Source: CAD feature listing. Evaluate the final solid. Frame: model axes, mm. A direction names the side the tool comes from. Coordinates: 2 decimals unless noted, no trailing zeros.
Item 1: Section query B-B, the plane z = 0. State how many separate pieces and enclosed holes the cut face has, then the cut area to 3 significant figures.
Item 2: Pull-direction query (Z, two-part tool) for faces 3 (the flat face through (44, 4, 26)), 4 (the flat face through (44, 4, -26)), 5 (the cylindrical face through (-36.926, 1.186, 22.404)); classes: +Z half, -Z half, draft (parallel to the pull), parting line (faces both ways), or undercut.
Item 3: Reachability of faces 1 (the cylindrical face through (-37.136, 1.214, -20.813)), 2 (the flat face through (38, 3.4, 24)) from +Z, -Z, +X, -X, +Y, -Y: full face, straight path, thin tool, end or side. Return the list, or none.
Item 4: Pin query (flat end, axial travel): pin 1 Ø15.5 at (x, z) = (-24, 1) entering from -Y; pin 2 Ø5 at (x, z) = (-40, 22) entering from +Y; pin 3 Ø9.5 at (x, z) = (-21, 0) entering from -Y; pin 4 Ø12 at (x, z) = (-23, 1) entering from -Y. Return the tip coordinate at first contact, or that it passes through.
Item 5: Line query: probe 1 along Z at (x, y) = (40, 2.75); probe 2 along Z at (x, y) = (40, 0.7); probe 3 along X at (y, z) = (3.45, 0). Output: solid intervals per line, ascending.
```python
from build123d import *

# Parameters (mm, degrees)
SKETCH1_W           = 96
SKETCH1_H           = 60
BOSS_EXTRUDE1_DEPTH = 8
CHAMFER1_SIZE       = 8
HOLE4_D             = 24.1
HOLE4_DEPTH         = 5.2
SKETCH10_R          = 10
CUT_EXTRUDE1_DEPTH  = 0.2
CHAMFER2_SIZE       = 0.2
SKETCH11_R          = 3.1
CUT_EXTRUDE2_DEPTH  = 2.2
CHAMFER3_SIZE       = 0.2
SKETCH15_R          = 8
CUT_EXTRUDE3_DEPTH  = 57.860882863
CHAMFER4_SIZE       = 0.4


# Read off the part's stored shape, not the designer's step: CBORE for M4 SHCS1, Sketch-Pattern1
with BuildPart() as part:
    # Sketch1 → Boss-Extrude1 (new body)
    with BuildSketch(Plane(origin=(0, 0, 0), x_dir=(1, 0, 0), z_dir=(0, 1, 0))):
        Rectangle(SKETCH1_W, SKETCH1_H)
    extrude(amount=BOSS_EXTRUDE1_DEPTH)

    # Chamfer1
    chamfer1_edges = [part.edges().sort_by_distance(p)[0] for p in [
        (48, 4, 30),
        (-48, 4, 30),
        (-48, 4, -30),
        (48, 4, -30),
    ]]
    chamfer(chamfer1_edges, length=CHAMFER1_SIZE)

    # Hole4
    with Locations(Plane(origin=(0, 0, 0), x_dir=(-1, 0, 0), z_dir=(0, -1, 0))):
        with Locations((21, 0), (-21, 0)):
            Hole(HOLE4_D / 2, depth=HOLE4_DEPTH)

    # CBORE for M4 SHCS1 outline → CBORE for M4 SHCS1 (revolve, cut)
    with BuildSketch(Plane(origin=(40, 0, 22), x_dir=(1, 0, 0), z_dir=(0, 0, 1))):
        Polygon((0, 0), (2.25, 0), (2.25, 3.4), (4, 3.4), (4, 7.975), (4.025, 8), (0, 8), align=None)
    revolve(axis=Axis((40, 0, 22), (0, 1, 0)), mode=Mode.SUBTRACT)

    # CBORE for M4 SHCS1 2 outline → CBORE for M4 SHCS1 2 (revolve, cut)
    with BuildSketch(Plane(origin=(-40, 0, -22), x_dir=(1, 0, 0), z_dir=(0, 0, 1))):
        Polygon((0, 8), (0, 0), (2.25, 0), (2.25, 3.4), (4, 3.4), (4, 7.975), (4.025, 8), align=None)
    revolve(axis=Axis((-40, 0, -22), (0, 1, 0)), mode=Mode.SUBTRACT)

    # CBORE for M4 SHCS1 3 outline → CBORE for M4 SHCS1 3 (revolve, cut)
    with BuildSketch(Plane(origin=(-40, 0, 22), x_dir=(1, 0, 0), z_dir=(0, 0, 1))):
        Polygon((0, 8), (0, 0), (2.25, 0), (2.25, 3.4), (4, 3.4), (4, 7.975), (4.025, 8), align=None)
    revolve(axis=Axis((-40, 0, 22), (0, 1, 0)), mode=Mode.SUBTRACT)

    # CBORE for M4 SHCS1 4 outline → CBORE for M4 SHCS1 4 (revolve, cut)
    with BuildSketch(Plane(origin=(40, 0, -22), x_dir=(1, 0, 0), z_dir=(0, 0, 1))):
        Polygon((0, 8), (0, 0), (2.25, 0), (2.25, 3.4), (4, 3.4), (4, 7.975), (4.025, 8), align=None)
    revolve(axis=Axis((40, 0, -22), (0, 1, 0)), mode=Mode.SUBTRACT)

    # Sketch10 → Cut-Extrude1 (cut)
    with BuildSketch(Plane.XZ.offset(-5.2)):
        with Locations(Location((-21, 0, 0), (0, 0, 270))):
            Circle(SKETCH10_R)
        with Locations(Location((21, 0, 0), (0, 0, 270))):
            Circle(SKETCH10_R)
    extrude(amount=-CUT_EXTRUDE1_DEPTH, mode=Mode.SUBTRACT)

    # Chamfer2
    chamfer2_edges = [part.edges().sort_by_distance(p)[0] for p in [
        (-33.05, 0, 0),
        (8.95, 0, 0),
        (-21, 5.4, 10),
        (21, 5.2, 10),
    ]]
    chamfer(chamfer2_edges, length=CHAMFER2_SIZE - 0.0001)  # a hair under: the kernel refuses the full size

    # Sketch11 → Cut-Extrude2 (cut)
    with BuildSketch(Plane.XZ):
        with Locations(Location((-40, 22, 0), (0, 0, 270))):
            Circle(SKETCH11_R)
    extrude(amount=-CUT_EXTRUDE2_DEPTH, mode=Mode.SUBTRACT)

    # Chamfer3
    chamfer3_edges = [part.edges().sort_by_distance(p)[0] for p in [
        (-40, 0, 25.1),
        (-42.25, 2.2, 22),
    ]]
    chamfer(chamfer3_edges, length=CHAMFER3_SIZE)

    # Sketch-Pattern1 outline → Sketch-Pattern1 (revolve, cut)
    with BuildSketch(Plane(origin=(40, 0, -22), x_dir=(1, 0, 0), z_dir=(0, 0, 1))):
        Polygon((3.1, 2.2), (2.25, 2.2), (2.25, 0), (3.3, 0), (3.1, 0.2), align=None)
    revolve(axis=Axis((40, 0, -22), (0, 1, 0)), mode=Mode.SUBTRACT)

    # Sketch-Pattern1 2 outline → Sketch-Pattern1 2 (revolve, cut)
    with BuildSketch(Plane(origin=(-40, 0, -22), x_dir=(1, 0, 0), z_dir=(0, 0, 1))):
        Polygon((3.1, 2.2), (2.25, 2.2), (2.25, 0), (3.3, 0), (3.1, 0.2), align=None)
    revolve(axis=Axis((-40, 0, -22), (0, 1, 0)), mode=Mode.SUBTRACT)

    # Sketch-Pattern1 3 outline → Sketch-Pattern1 3 (revolve, cut)
    with BuildSketch(Plane(origin=(40, 0, 22), x_dir=(1, 0, 0), z_dir=(0, 0, 1))):
        Polygon((3.1, 2.2), (2.25, 2.2), (2.25, 0), (3.3, 0), (3.1, 0.2), align=None)
    revolve(axis=Axis((40, 0, 22), (0, 1, 0)), mode=Mode.SUBTRACT)

    # Sketch15 → Cut-Extrude3 (cut, through all)
    with BuildSketch(Plane.XZ.offset(-5.4)):
        with Locations(Location((-21, 0, 0), (0, 0, 270))):
            Circle(SKETCH15_R)
        with Locations(Location((21, 0, 0), (0, 0, 270))):
            Circle(SKETCH15_R)
    extrude(amount=-CUT_EXTRUDE3_DEPTH, mode=Mode.SUBTRACT)

    # Chamfer4
    chamfer4_edges = [part.edges().sort_by_distance(p)[0] for p in [
        (-21, 8, 8),
        (-21, 5.4, 8),
        (21, 8, 8),
        (21, 5.4, 8),
    ]]
    chamfer(chamfer4_edges, length=CHAMFER4_SIZE)


solid = part.part
```
Verdict:
1. separate pieces: 3
1. enclosed holes: 0
1. area: 425 mm2
2. face 3: +Z half
2. face 4: -Z half
2. face 5: undercut
3. face 1: -Y
3. face 2: +Y
4. pin 1: stops at y = 5.2
4. pin 2: stops at y = 3.4
4. pin 3: passes through
4. pin 4: stops at y = 5.56
5. probe 1: z = -30 to -24.25, -19.75 to 19.75, 24.25 to 30
5. probe 2: z = -30 to -25.1, -18.9 to 18.9, 25.1 to 30
5. probe 3: x = -48 to -33.05, -8.95 to 8.95, 33.05 to 48
